Here's how the part is built. I have some questions about the finished solid (model axes, mm). Give positions to 0.01 mm unless a question says otherwise; leave off trailing zeros. Order: outer loops, then holes, each group sorted by start corner. A loop starts at its lowest first (then second) coordinate and runs counter-clockwise, first axis right, second up.
from build123d import *

# Parameters (mm, degrees)
SKETCH2_R           = 20
BOSS_EXTRUDE1_DEPTH = 420
SKETCH3_W           = 5
SKETCH3_H           = 2
SKETCH4_W           = 2
SKETCH4_H           = 1.5
CUT_EXTRUDE2_DEPTH  = 30


with BuildPart() as part:
    # Sketch2 → Boss-Extrude1 (new body)
    with BuildSketch(Plane(origin=(0, 0, 0), x_dir=(1, 0, 0), z_dir=(0, 1, 0))):
        Circle(SKETCH2_R)
    extrude(amount=BOSS_EXTRUDE1_DEPTH)

    # Sketch3 → Cut-Revolve1 (revolve, cut)
    with BuildSketch(Plane(origin=(0, 0, 0), x_dir=(0, 0, -1), z_dir=(1, 0, 0))):
        with Locations((17.5, 9)):
            Rectangle(SKETCH3_W, SKETCH3_H)
    revolve(axis=Axis((0, 0, 0), (0, 1, 0)), mode=Mode.SUBTRACT)

    # Sketch4 → Cut-Extrude2 (cut)
    with BuildSketch(Plane(origin=(0, 420, 0), x_dir=(1, 0, 0), z_dir=(0, 1, 0))):
        with Locations((0, 19.25)):
            Rectangle(SKETCH4_W, SKETCH4_H)
    extrude(amount=-CUT_EXTRUDE2_DEPTH, mode=Mode.SUBTRACT)


solid = part.part
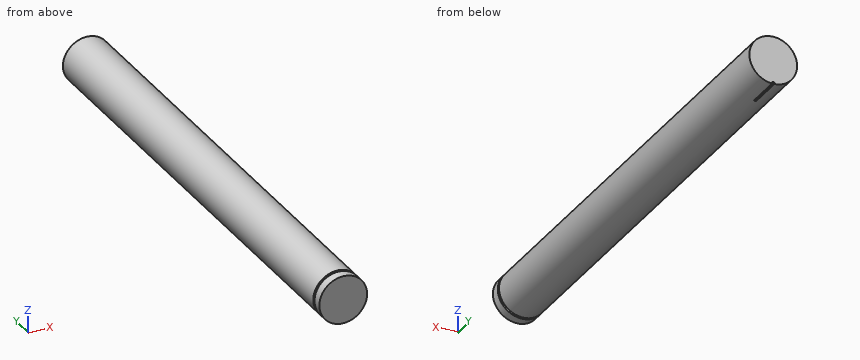
Q1. If we section it at A-A on z = 9: List the corners of the cut face in (x, y) for me, plus the area to 3 significant figures.
Filled sheet:
outline: (-17.86, 0) - (17.86, 0) - (17.86, 8) - (12, 8) - (12, 10) - (17.86, 10) - (17.86, 420) - (-17.86, 420) - (-17.86, 10) - (-12, 10) - (-12, 8) - (-17.86, 8) - close
area: 15,000 mm2
Q2. I'm going to push flat-ended pins straight in: P1, Ø1.2, axis at y = 406.5, z = -19, coming from the +X side; P2, Ø1.2, axis at y = 398.5, z = -19, coming from the -X side; P3, Ø0.6, axis at x = 0, y = 406.5, coming from the -Z side. Where does each tip first touch, or does it pass through?
Filled sheet:
P1: stops at x = 7.84
P2: stops at x = -7.84
P3: stops at z = -18.5
Q3. If we section it at B-B on x = -5.5: List the corners of the cut face in (y, z) for me.
Filled sheet:
outline: (0, -19.23) - (8, -19.23) - (8, -13.96) - (10, -13.96) - (10, -19.23) - (420, -19.23) - (420, 19.23) - (10, 19.23) - (10, 13.96) - (8, 13.96) - (8, 19.23) - (0, 19.23) - close
Q4. If we section it at C-C on y = 206.5: List the corners of the cut face in (x, z) for me.
Filled sheet:
outline: circle Ø40 at (0, 0)
Q5. I need wall thicknesses on L1, parallel to Y at x = -6, z = 18; L2, parallel to Z at x = -1, y = 48.5; L3, parallel to X at y = 216.5, z = 1.5. Which ranges of each line are inside material? Lowest first, please.
Filled sheet:
L1: y = 0 to 8, 10 to 420
L2: z = -19.97 to 19.97
L3: x = -19.94 to 19.94
